```python
from build123d import *

# Parameters (mm, degrees)
F0_W         = 19.62069033
F0_H         = 25.4568966
F1_DEPTH     = 5.4
F2_SIZE      = 5
F3_SIZE      = 5
F4_W         = 22.1276450902
F4_H         = 1.5373004135
F5_DEPTH     = 0.2
F7_DEPTH     = 25.5
F8_W         = 23.348543793
F8_H         = 5.9792976826
F9_DEPTH     = 1.7
F10_R        = 2
F11_T1_DEPTH = 28.4568966
F11_T3_DEPTH = 8.8
F11_T6_ANGLE = 90
F12_T1_DEPTH = 22.62069033
F12_T3_DEPTH = 8.8
F12_T6_ANGLE = 90.0000000053
F14_DEPTH    = 5.6
F15_W        = 9.62069033
F15_H        = 12.3144993559
F16_DEPTH    = 0.1


# Not quite as in the source:
# - a fillet or chamfer that OpenCascade refuses, or shapes differently, is made with other operations: its cross-section is extruded or revolved along the edge and cut away or added


with BuildPart() as f1:
    # F0 (on Top) → F1 (new body, symmetric)
    with BuildSketch(Plane.XY):
        Rectangle(F0_W, F0_H)
    extrude(amount=F1_DEPTH, both=True)

    # F2
    f2_edges = [f1.edges().sort_by_distance(p)[0] for p in [
        (-9.810345, 0, 5.4),
    ]]
    chamfer(f2_edges, length=F2_SIZE)

    # F3
    f3_edges = [f1.edges().sort_by_distance(p)[0] for p in [
        (9.810345, 0, 5.4),
    ]]
    chamfer(f3_edges, length=F3_SIZE)

    # F4 (on face) → F5 (join)
    with BuildSketch(Plane(origin=(5.1051725825, 0, 5.1051725825), x_dir=(0, 1, 0), z_dir=(0.7071067812, 0, 0.7071067812))):
        with Locations((0.2083815634, -0.7686502067)):
            Rectangle(F4_W, F4_H)
        Polygon((11.2722041085, -2.2796541452), (-10.8554409817, -2.2294183727), (-10.8554409817, -3.5751299001), (11.2722041085, -3.5751299001), align=None)
        Polygon((11.2722041085, -4.2798109353), (-10.8554409817, -4.4601280242), (-10.8554409817, -5.5370246992), (11.2722041085, -5.5370246992), align=None)
    extrude(amount=F5_DEPTH)

    # F6 (on face) → F7 (cut)
    with BuildSketch(Plane.XZ.offset(12.7284483)):
        Polygon((4.140063189, 4.6230903827), (-3.1588820275, 4.6230903827), (-7.9239970073, 0.6864351453), (7.2048916481, 0.6864351453), align=None)
    extrude(amount=-F7_DEPTH, mode=Mode.SUBTRACT)

    # F8 (on face) → F9 (cut)
    with BuildSketch(Plane(origin=(-5.1051725825, 0, 5.1051725825), x_dir=(0, -1, 0), z_dir=(-0.7071067812, 0, 0.7071067812))):
        with Locations((-0.0411020592, -2.9896488413)):
            Rectangle(F8_W, F8_H)
    extrude(amount=-F9_DEPTH, mode=Mode.SUBTRACT)

    # F10
    f10_edges = [f1.edges().sort_by_distance(p)[0] for p in [
        (0, -12.728448, -5.4),
    ]]
    fillet(f10_edges, radius=F10_R)

    # F11: fillet of radius 2 on 1 edges, made by hand

    # F11_s2 → F11_t1 (cut)
    with BuildSketch(Plane.XZ.offset(-17.7284483)):
        with BuildLine():
            ThreePointArc((-7.810345165, -5.4), (-9.2245587274, -4.8142135624), (-9.810345165, -3.4))
            Line((-9.810345165, -3.4), (-9.810345165, -5.4))
            Line((-9.810345165, -5.4), (-7.810345165, -5.4))
        make_face()
    extrude(amount=F11_T1_DEPTH, mode=Mode.SUBTRACT)

    # F11_s4 → F11_t3 (cut)
    with BuildSketch(Plane.XY.offset(-3.4)):
        with BuildLine():
            ThreePointArc((-7.810345165, -12.7284483), (-9.2245587274, -12.1426618624), (-9.810345165, -10.7284483))
            Line((-9.810345165, -10.7284483), (-9.810345165, -12.7284483))
            Line((-9.810345165, -12.7284483), (-7.810345165, -12.7284483))
        make_face()
    extrude(amount=F11_T3_DEPTH, mode=Mode.SUBTRACT)

    # F11_s5 → F11_t6 (revolve, cut)
    with BuildSketch(Plane.XZ.offset(10.7284483)):
        with BuildLine():
            ThreePointArc((-7.810345165, -5.4), (-9.2245587274, -4.8142135624), (-9.810345165, -3.4))
            Line((-9.810345165, -3.4), (-9.810345165, -5.4))
            Line((-9.810345165, -5.4), (-7.810345165, -5.4))
        make_face()
    revolve(axis=Axis((-9.810345165, -10.7284483, -3.4), (-1, 0, 0)), revolution_arc=F11_T6_ANGLE, mode=Mode.SUBTRACT)

    # F12: fillet of radius 2 on 1 edges, made by hand

    # F12_s2 → F12_t1 (cut)
    with BuildSketch(Plane.YZ.offset(-7.810345165)):
        with BuildLine():
            ThreePointArc((10.7284483, -5.4), (12.1426618624, -4.8142135624), (12.7284483, -3.4))
            Line((12.7284483, -3.4), (12.7284483, -5.4))
            Line((12.7284483, -5.4), (10.7284483, -5.4))
        make_face()
    extrude(amount=F12_T1_DEPTH, mode=Mode.SUBTRACT)

    # F12_s4 → F12_t3 (cut)
    with BuildSketch(Plane.XY.offset(-3.4)):
        with BuildLine():
            ThreePointArc((-7.810345165, 12.7284483), (-9.2245587274, 12.1426618624), (-9.810345165, 10.7284483))
            Line((-9.810345165, 10.7284483), (-9.810345165, 12.7284483))
            Line((-9.810345165, 12.7284483), (-7.810345165, 12.7284483))
        make_face()
    extrude(amount=F12_T3_DEPTH, mode=Mode.SUBTRACT)

    # F12_s5 → F12_t6 (revolve, cut)
    with BuildSketch(Plane.YZ.offset(-7.8103451651)):
        with BuildLine():
            ThreePointArc((12.7284483, -3.4), (12.1426618624, -4.8142135624), (10.7284483, -5.4))
            Line((10.7284483, -5.4), (12.7284483, -5.4))
            Line((12.7284483, -5.4), (12.7284483, -3.4))
        make_face()
    revolve(axis=Axis((-7.8103451651, 12.7284483, -3.4000000001), (0, 1, 0)), revolution_arc=F12_T6_ANGLE, mode=Mode.SUBTRACT)

    # F13 (on face) → F14 (cut)
    with BuildSketch(Plane.XY.offset(0.6864351453)):
        Polygon((6.1108670197, -10.853772983), (6.3247303478, 11.9756069034), (-5.7491413318, 11.2674161792), (-5.7491413318, -10.853772983), align=None)
    extrude(amount=-F14_DEPTH, mode=Mode.SUBTRACT)

    # F15 (on face) → F16 (cut)
    with BuildSketch(Plane.XY.offset(5.4)):
        with Locations((0, -0.4627322778)):
            Rectangle(F15_W, F15_H)
    extrude(amount=-F16_DEPTH, mode=Mode.SUBTRACT)


solid = f1.part
```
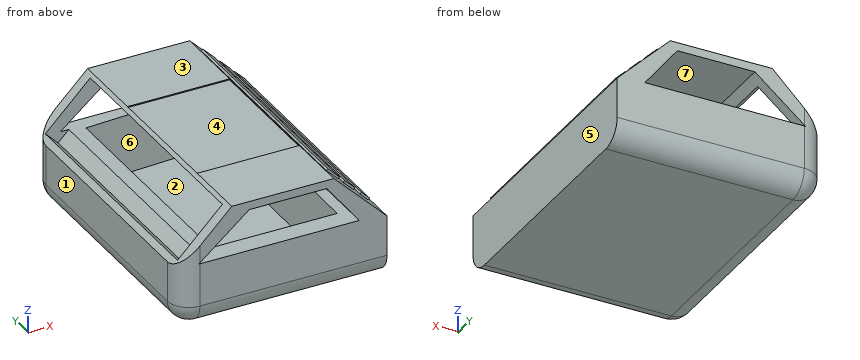
Check sheet for the modelled part. Datum: model origin and axes. Units: mm. Face numbers are marked on the shaded views. A direction names the side the tool comes from. Give positions to 0.01 mm unless a question says otherwise; leave off trailing zeros. Order: outer loops, then holes, each group sorted by start corner. A loop starts at its lowest first (then second) coordinate and runs counter-clockwise, first axis right, second up. Notation, with made-up numbers: (13, -22.5) -> (57, -22.5) arc R16 cw to (57, 0.5) -> close; hole circle Ø3 at (72.25, -31.75). An arc over 180 degrees is marked (long way). Use CSV: the item, a comma, the result in double quotes. Start each with the question number.
1) Sectioned sample at D-D, the plane x = 3. Record the boundary of the cut face in (y, z), plus the area to 3 significant figures.
2) Go/stop test with flat-tipped pins: P1, Ø1.5, axis at x = 6.5, y = 1, coming from the +Z side; P2, Ø2, axis at y = -0.5, z = 1.5, coming from the +X side; P3, Ø3, axis at y = -1.5, z = 3.5, coming from the -X side. Record where each tip stops, or that it passes through.
3) Material ranges on line 1 (X direction, y = -3, z = -3.5); line 2 (Z direction, x = -1.25, y = 1.5); line 3 (Z direction, x = 4, y = -9.5), recorded low to high. Write a range as from..to.
4) Sectioned sample at B-B, the plane x = -1.25. Record the boundary of the cut face in (y, z), plus the area to 3 significant figures.
5) Set-up check for the marked faces 4, 5, 6 and 7: record each of +Z, -Z, +X, -X, +Y, -Y from which the full face is reachable in a straight line by a thin tool's end or side.
6) Mould release check, pull along Z, two halves, no side actions. Record for the marked faces 1, 2 and 3: released by +Z, released by -Z, zero draft, split by the parting line, or undercut.
7) Sectioned sample at A-A, the plane z = -3. Record the boundary of the cut face in (x, y).
Recorded:
1,outline,"(-12.73, -3.4) arc R2 ccw to (-10.73, -5.4) -> (10.73, -5.4) arc R2 ccw to (12.73, -3.4) -> (12.73, 0.69) -> (11.78, 0.69) -> (11.78, -4.91) -> (-10.85, -4.91) -> (-10.85, 0.69) -> (-12.73, 0.69) -> close; (-12.73, 4.62) -> (12.73, 4.62) -> (12.73, 5.4) -> (5.69, 5.4) -> (5.69, 5.3) -> (-6.62, 5.3) -> (-6.62, 5.4) -> (-12.73, 5.4) -> close"
1,area,"45.0 mm2"
2,P1,"z = 4.74"
2,P2,"x = 9.71"
2,P3,"x = -5"
3,line 1,"-9.81..-5.75, 6.18..9.81"
3,line 2,"-5.4..-4.91, 4.62..5.3"
3,line 3,"-5.4..-4.91, 4.62..5.4"
4,outline,"(-12.73, -3.4) arc R2 ccw to (-10.73, -5.4) -> (10.73, -5.4) arc R2 ccw to (12.73, -3.4) -> (12.73, 0.69) -> (11.53, 0.69) -> (11.53, -4.91) -> (-10.85, -4.91) -> (-10.85, 0.69) -> (-12.73, 0.69) -> close; (-12.73, 4.62) -> (12.73, 4.62) -> (12.73, 5.4) -> (5.69, 5.4) -> (5.69, 5.3) -> (-6.62, 5.3) -> (-6.62, 5.4) -> (-12.73, 5.4) -> close"
4,area,"46.4 mm2"
5,face 4,"+Z"
5,face 5,"+Z, -Z, +X, +Y, -Y"
5,face 6,"none"
5,face 7,"+Y, -Y"
6,face 1,"zero draft"
6,face 2,"undercut"
6,face 3,"released by +Z"
7,outline,"(-9.81, -10.73) arc R2 ccw to (-7.81, -12.73) -> (9.81, -12.73) -> (9.81, 12.73) -> (-7.81, 12.73) arc R2 ccw to (-9.81, 10.73) -> close; hole (-5.75, -10.85) -> (6.11, -10.85) -> (6.32, 11.98) -> (-5.75, 11.27) -> close"
